```python
from build123d import *

# Parameters (mm, degrees)
F0_R         = 21
F1_DEPTH     = 5.5
F2_R         = 22
F3_DEPTH     = 2
F4_R         = 22
F5_DEPTH     = 2
F7_DEPTH     = 15.001
F8_R         = 18.5
F8_R_2       = 4
F9_DEPTH     = 10
F11_DEPTH    = 5.001
F12_T1_DEPTH = 5


# Not quite as in the source:
# - a fillet or chamfer that OpenCascade refuses, or shapes differently, is made with other operations: its cross-section is extruded or revolved along the edge and cut away or added


with BuildPart() as f1:
    # F0 (on Right) → F1 (new body, symmetric)
    with BuildSketch(Plane.YZ):
        Circle(F0_R)
    extrude(amount=F1_DEPTH, both=True)

    # F2 (on face) → F3 (join)
    with BuildSketch(Plane.YZ.offset(5.5)):
        Circle(F2_R)
    extrude(amount=F3_DEPTH)

    # F4 (on face) → F5 (join)
    with BuildSketch(Plane(origin=(-5.5, 0, 0), x_dir=(0, -1, 0), z_dir=(-1, 0, 0))):
        Circle(F4_R)
    extrude(amount=F5_DEPTH)

    # F6 (on face) → F7 (cut, through all)
    with BuildSketch(Plane(origin=(-7.5, 0, 0), x_dir=(0, -1, 0), z_dir=(-1, 0, 0))):
        with BuildLine():
            Line((-1.5, -2), (1.5, -2))
            ThreePointArc((1.5, -2), (0, 2.5), (-1.5, -2))
        make_face()
    extrude(amount=-F7_DEPTH, mode=Mode.SUBTRACT)

    # F8 (on face) → F9 (cut)
    with BuildSketch(Plane.YZ.offset(7.5)):
        Circle(F8_R)
        Circle(F8_R_2, mode=Mode.SUBTRACT)
    extrude(amount=-F9_DEPTH, mode=Mode.SUBTRACT)

    # F10 (on face) → F11 (cut, through all)
    with BuildSketch(Plane.YZ.offset(-2.5)):
        with BuildLine():
            Line((4.7881523344, 17.8696277863), (1.2940952255, 4.8296291314))
            ThreePointArc((1.2940952255, 4.8296291314), (2.5827855501, 3.5548993357), (4.1933528397, 2.7231951751))
            Line((4.1933528397, 2.7231951751), (15.515405507, 10.0758221478))
            ThreePointArc((15.515405507, 10.0758221478), (10.8740271674, 14.9668143959), (4.7881523344, 17.8696277863))
        make_face()
        with BuildLine():
            ThreePointArc((4.9931476738, 0.2616797812), (4.1790348058, -1.3578507196), (3.8857298073, -3.1466019552))
            Line((3.8857298073, -3.1466019552), (14.377200287, -11.6424272344))
            ThreePointArc((14.377200287, -11.6424272344), (17.5945455515, -5.7168143959), (18.474646393, 0.9682151905))
            Line((18.474646393, 0.9682151905), (4.9931476738, 0.2616797812))
        make_face()
        with BuildLine():
            ThreePointArc((1.7918397477, -4.6679021325), (0, -4.3940972321), (-1.7918397477, -4.6679021325))
            Line((-1.7918397477, -4.6679021325), (-6.6298070666, -17.2712378902))
            ThreePointArc((-6.6298070666, -17.2712378902), (0, -18.5), (6.6298070666, -17.2712378902))
            Line((6.6298070666, -17.2712378902), (1.7918397477, -4.6679021325))
        make_face()
        with BuildLine():
            ThreePointArc((-3.8857298073, -3.1466019552), (-4.1790348058, -1.3578507196), (-4.9931476738, 0.2616797812))
            Line((-4.9931476738, 0.2616797812), (-18.474646393, 0.9682151905))
            ThreePointArc((-18.474646393, 0.9682151905), (-17.5945455515, -5.7168143959), (-14.377200287, -11.6424272344))
            Line((-14.377200287, -11.6424272344), (-3.8857298073, -3.1466019552))
        make_face()
        with BuildLine():
            ThreePointArc((-4.1933528397, 2.7231951751), (-2.5827855501, 3.5548993357), (-1.2940952255, 4.8296291314))
            Line((-1.2940952255, 4.8296291314), (-4.7881523344, 17.8696277863))
            ThreePointArc((-4.7881523344, 17.8696277863), (-10.8740271674, 14.9668143959), (-15.515405507, 10.0758221478))
            Line((-15.515405507, 10.0758221478), (-4.1933528397, 2.7231951751))
        make_face()
    extrude(amount=-F11_DEPTH, mode=Mode.SUBTRACT)

    # F12: fillet of radius 1 on 20 edges, made by hand

    # F12_s2 → F12_t1 (join)
    with BuildSketch(Plane.YZ.offset(-7.5)):
        with BuildLine():
            ThreePointArc((4.6223226532, 3.0017714292), (4.1563467345, 2.8435407412), (3.671320929, 2.9267301361))
            ThreePointArc((3.671320929, 2.9267301361), (3.9299597122, 2.8188656209), (4.1933528397, 2.7231951751))
            Line((4.1933528397, 2.7231951751), (4.6223226532, 3.0017714292))
        make_face()
        with BuildLine():
            ThreePointArc((1.4264780248, 5.3236884645), (1.4199861758, 4.831623059), (1.6489852086, 4.3960430429))
            ThreePointArc((1.6489852086, 4.3960430429), (1.466476179, 4.6086911748), (1.2940952255, 4.8296291314))
            Line((1.2940952255, 4.8296291314), (1.4264780248, 5.3236884645))
        make_face()
        with BuildLine():
            ThreePointArc((14.65275333, 9.5156092737), (15.0918050058, 10.1744115971), (14.9142922547, 10.9459529755))
            ThreePointArc((14.9142922547, 10.9459529755), (15.221067912, 10.5151838604), (15.515405507, 10.0758221478))
            Line((15.515405507, 10.0758221478), (14.65275333, 9.5156092737))
        make_face()
        with BuildLine():
            ThreePointArc((4.521932413, 16.8760815136), (5.0128162263, 17.4972255847), (5.8014501386, 17.5668203238))
            ThreePointArc((5.8014501386, 17.5668203238), (5.2969654732, 17.7254663345), (4.7881523344, 17.8696277863))
            Line((4.7881523344, 17.8696277863), (4.521932413, 16.8760815136))
        make_face()
        with BuildLine():
            ThreePointArc((5.5039345567, 0.2884489874), (5.0339464546, 0.1425665301), (4.6904498348, -0.2098261196))
            ThreePointArc((4.6904498348, -0.2098261196), (4.8362918345, 0.0294621688), (4.9931476738, 0.2616797812))
            Line((4.9931476738, 0.2616797812), (5.5039345567, 0.2884489874))
        make_face()
        with BuildLine():
            ThreePointArc((4.2832305314, -3.4684916949), (3.9887497267, -3.0742182326), (3.9179863263, -2.5872243429))
            ThreePointArc((3.9179863263, -2.5872243429), (3.8953248556, -2.8665364113), (3.8857298073, -3.1466019552))
            Line((3.8857298073, -3.1466019552), (4.2832305314, -3.4684916949))
        make_face()
        with BuildLine():
            ThreePointArc((1.2498722119, -4.5257227166), (1.6911638308, -4.7435120977), (1.9751406031, -5.1454171863))
            Line((1.9751406031, -5.1454171863), (1.7918397477, -4.6679021325))
            ThreePointArc((1.7918397477, -4.6679021325), (1.5225165542, -4.5904825531), (1.2498722119, -4.5257227166))
        make_face()
        with BuildLine():
            ThreePointArc((-1.9751406031, -5.1454171863), (-1.6911638308, -4.7435120977), (-1.2498722119, -4.5257227166))
            ThreePointArc((-1.2498722119, -4.5257227166), (-1.5225165542, -4.5904825531), (-1.7918397477, -4.6679021325))
            Line((-1.7918397477, -4.6679021325), (-1.9751406031, -5.1454171863))
        make_face()
        with BuildLine():
            ThreePointArc((-5.5039345567, 0.2884489874), (-5.0339464546, 0.1425665301), (-4.6904498348, -0.2098261196))
            ThreePointArc((-4.6904498348, -0.2098261196), (-4.8362918345, 0.0294621688), (-4.9931476738, 0.2616797812))
            Line((-4.9931476738, 0.2616797812), (-5.5039345567, 0.2884489874))
        make_face()
        with BuildLine():
            ThreePointArc((-3.9179863263, -2.5872243429), (-3.9887497267, -3.0742182326), (-4.2832305314, -3.4684916949))
            Line((-4.2832305314, -3.4684916949), (-3.8857298073, -3.1466019552))
            ThreePointArc((-3.8857298073, -3.1466019552), (-3.8953248556, -2.8665364113), (-3.9179863263, -2.5872243429))
        make_face()
        with BuildLine():
            ThreePointArc((-3.671320929, 2.9267301361), (-4.1563467345, 2.8435407412), (-4.6223226532, 3.0017714292))
            Line((-4.6223226532, 3.0017714292), (-4.1933528397, 2.7231951751))
            ThreePointArc((-4.1933528397, 2.7231951751), (-3.9299597122, 2.8188656209), (-3.671320929, 2.9267301361))
        make_face()
        with BuildLine():
            ThreePointArc((-1.4264780248, 5.3236884645), (-1.4199861758, 4.831623059), (-1.6489852086, 4.3960430429))
            ThreePointArc((-1.6489852086, 4.3960430429), (-1.466476179, 4.6086911748), (-1.2940952255, 4.8296291314))
            Line((-1.2940952255, 4.8296291314), (-1.4264780248, 5.3236884645))
        make_face()
        with BuildLine():
            ThreePointArc((13.5778319997, -10.9951115587), (14.3400646715, -11.2090934022), (15.0189896702, -10.8018493457))
            ThreePointArc((15.0189896702, -10.8018493457), (14.7041027879, -11.2267253108), (14.377200287, -11.6424272344))
            Line((14.377200287, -11.6424272344), (13.5778319997, -10.9951115587))
        make_face()
        with BuildLine():
            ThreePointArc((17.447461256, 0.9143826986), (18.189895813, 0.639468523), (18.4997856244, -0.0890609411))
            ThreePointArc((18.4997856244, -0.0890609411), (18.4947726116, 0.4397568007), (18.474646393, 0.9682151905))
            Line((18.474646393, 0.9682151905), (17.447461256, 0.9143826986))
        make_face()
        with BuildLine():
            ThreePointArc((6.2611916607, -16.3109619271), (6.229157638, -17.1020123027), (5.6320461618, -17.6218630125))
            ThreePointArc((5.6320461618, -17.6218630125), (6.133432615, -17.4536816849), (6.6298070666, -17.2712378902))
            Line((6.6298070666, -17.2712378902), (6.2611916607, -16.3109619271))
        make_face()
        with BuildLine():
            ThreePointArc((-6.2611916607, -16.3109619271), (-6.229157638, -17.1020123027), (-5.6320461618, -17.6218630125))
            ThreePointArc((-5.6320461618, -17.6218630125), (-6.133432615, -17.4536816849), (-6.6298070666, -17.2712378902))
            Line((-6.6298070666, -17.2712378902), (-6.2611916607, -16.3109619271))
        make_face()
        with BuildLine():
            ThreePointArc((-17.447461256, 0.9143826986), (-18.189895813, 0.639468523), (-18.4997856244, -0.0890609411))
            ThreePointArc((-18.4997856244, -0.0890609411), (-18.4947726116, 0.4397568007), (-18.474646393, 0.9682151905))
            Line((-18.474646393, 0.9682151905), (-17.447461256, 0.9143826986))
        make_face()
        with BuildLine():
            ThreePointArc((-13.5778319997, -10.9951115587), (-14.3400646715, -11.2090934022), (-15.0189896702, -10.8018493457))
            ThreePointArc((-15.0189896702, -10.8018493457), (-14.7041027879, -11.2267253108), (-14.377200287, -11.6424272344))
            Line((-14.377200287, -11.6424272344), (-13.5778319997, -10.9951115587))
        make_face()
        with BuildLine():
            ThreePointArc((-4.521932413, 16.8760815136), (-5.0128162263, 17.4972255847), (-5.8014501386, 17.5668203238))
            ThreePointArc((-5.8014501386, 17.5668203238), (-5.2969654732, 17.7254663345), (-4.7881523344, 17.8696277863))
            Line((-4.7881523344, 17.8696277863), (-4.521932413, 16.8760815136))
        make_face()
        with BuildLine():
            ThreePointArc((-14.65275333, 9.5156092737), (-15.0918050058, 10.1744115971), (-14.9142922547, 10.9459529755))
            ThreePointArc((-14.9142922547, 10.9459529755), (-15.221067912, 10.5151838604), (-15.515405507, 10.0758221478))
            Line((-15.515405507, 10.0758221478), (-14.65275333, 9.5156092737))
        make_face()
    extrude(amount=F12_T1_DEPTH)


solid = f1.part
```
For this review, take the finished solid that the model builds, in its own axes (mm). Coordinates: 2 decimals unless noted, no trailing zeros. Write each loop counter-clockwise with the first axis right and the second up, starting at its lowest first coordinate (ties: lowest second). Pieces come first, ordered by that corner, then holes. Notation, with made-up numbers: (68.5, 3.5) - (118.5, 3.5) arc R15 cw to (118.5, 22.5) - close; hole circle Ø3 at (67, 68.5). An arc over 180 degrees is marked (long way). Answer in a Markdown table with one row per item. Add a question column.
Q1. We need section D-D, the plane z = 9. State the section outline as (x, y) points, and give its area (3 significant figures).
Q2. For probe 1 along Z at (x, y) = (0.75, 0); probe 2 along Y at (x, z) = (-1.75, 1.5); probe 3 along Y at (x, z) = (-3.75, -11), list the stretches that pass through material, from the lowest coordinate up.
Q3. Draft analysis for pull direction X (two halves, no side actions). For faces 1 (the flat face through (7.5, -5, 18)), 2 (the flat face through (-4.96, -4.09, -10.65)), 3 (the cylindrical face through (0.08, 20.03, 6.31)), state which applies: +X half, -X half, draft (parallel to the pull), parting line (faces both ways), or undercut.
Q4. We need section A-A, the plane y = 0. State the section outline as (x, z) points.
Q5. We need section B-B, the plane x = 6.25. State the section outline as (y, z) points.
Q6. We need section C-C, the plane z = -9. State the section outline as (x, y) points.
Q7. For P1, Ø3, axis at x = -4.5, z = 5, coming from the +Y side; P2, Ø4, axis at y = 10, z = 5, coming from the +X side; P3, Ø1.5, axis at y = 0, z = -1, coming from the +X side; P4, Ø0.9, axis at x = -2, y = 0.5, coming from the +Z side, all flat-tipped, find the tip position at first contact; note any pin that passes through.
Answer list:
| question | item | result |
|---|---|---|
| 1 | outline | (-7.5, -20.07) - (-5.5, -20.07) - (-5.5, -18.97) - (5.5, -18.97) - (5.5, -20.07) - (7.5, -20.07) - (7.5, -16.16) - (-2.5, -16.16) - (-2.5, -13.86) - (-7.5, -13.86) - close; (-7.5, -2.41) - (-2.5, -2.41) - (-2.5, 2.41) - (-7.5, 2.41) - close; (-7.5, 13.86) - (-2.5, 13.86) - (-2.5, 16.16) - (7.5, 16.16) - (7.5, 20.07) - (5.5, 20.07) - (5.5, 18.97) - (-5.5, 18.97) - (-5.5, 20.07) - (-7.5, 20.07) - close |
| 1 | area | 140 mm2 |
| 2 | probe 1 | z = -21 to -18.5, -4 to -2, 2.5 to 4, 18.5 to 21 |
| 2 | probe 2 | y = -20.95 to -18.44, -3.71 to -2, 2 to 3.71, 18.44 to 20.95 |
| 2 | probe 3 | y = -17.89 to -14.83, -13.58 to -4.22, 4.22 to 13.58, 14.83 to 17.89 |
| 3 | face 1 | +X half |
| 3 | face 2 | draft |
| 3 | face 3 | undercut |
| 4 | outline | (-7.5, -22) - (-5.5, -22) - (-5.5, -21) - (5.5, -21) - (5.5, -22) - (7.5, -22) - (7.5, -18.5) - (-7.5, -18.5) - close; (-7.5, -4.39) - (-2.5, -4.39) - (-2.5, -4) - (7.5, -4) - (7.5, -2) - (-7.5, -2) - close; (-7.5, 2.5) - (7.5, 2.5) - (7.5, 4) - (-2.5, 4) - (-2.5, 18.5) - (7.5, 18.5) - (7.5, 22) - (5.5, 22) - (5.5, 21) - (-5.5, 21) - (-5.5, 22) - (-7.5, 22) - close |
| 5 | outline | circle Ø44 at (0, 0); circle Ø8 at (0, 0); hole circle Ø37 at (0, 0); hole (-1.5, -2) - (1.5, -2) arc R2.5 ccw (long way) to start |
| 6 | outline | (-7.5, -20.07) - (-5.5, -20.07) - (-5.5, -18.97) - (5.5, -18.97) - (5.5, -20.07) - (7.5, -20.07) - (7.5, -16.16) - (-7.5, -16.16) - close; (-7.5, -11.11) - (-2.5, -11.11) - (-2.5, -3.45) - (-7.5, -3.45) - close; (-7.5, 3.45) - (-2.5, 3.45) - (-2.5, 11.11) - (-7.5, 11.11) - close; (-7.5, 16.16) - (7.5, 16.16) - (7.5, 20.07) - (5.5, 20.07) - (5.5, 18.97) - (-5.5, 18.97) - (-5.5, 20.07) - (-7.5, 20.07) - close |
| 7 | P1 | stops at y = 21.65 |
| 7 | P2 | stops at x = -2.5 |
| 7 | P3 | passes through |
| 7 | P4 | stops at z = 21 |
